The model under review builds one solid part; all positions refer to its coordinate system, in mm. A direction names the side the tool comes from. Round coordinates to 2 decimals unless told otherwise and drop trailing zeros. Write each loop counter-clockwise with the first axis right and the second up, starting at its lowest first coordinate (ties: lowest second). Pieces come first, ordered by that corner, then holes. Notation, with made-up numbers: (38.25, 8.5) - (85.25, 8.5) arc R32 cw to (85.25, 47.5) - close; hole circle Ø10 at (56.25, -1.75). An arc over 180 degrees is marked (long way). Write each question's results on one line, items separated by ' | '.
```python
from build123d import *

# Parameters (mm, degrees)
BOSS_EXTRUDE1_DEPTH = 15
SKETCH2_R           = 20
BOSS_EXTRUDE2_DEPTH = 25
SKETCH3_R           = 12.5
CUT_EXTRUDE1_DEPTH  = 103.220350224
SKETCH4_W           = 15
SKETCH4_H           = 65
BOSS_EXTRUDE3_DEPTH = 15


with BuildPart() as part:
    # Sketch1 → Boss-Extrude1 (new body)
    with BuildSketch(Plane.XY):
        with BuildLine():
            Line((0, 0), (68, 0))
            Line((68, 0), (68, 65))
            Line((68, 65), (0, 65))
            ThreePointArc((0, 65), (-32.5, 32.5), (0, 0))
        make_face()
    extrude(amount=BOSS_EXTRUDE1_DEPTH)

    # Sketch2 → Boss-Extrude2 (add)
    with BuildSketch(Plane.XY.offset(15)):
        with Locations((0, 32.5)):
            Circle(SKETCH2_R)
    extrude(amount=BOSS_EXTRUDE2_DEPTH)

    # Sketch3 → Cut-Extrude1 (cut, through all)
    with BuildSketch(Plane.XY.offset(40)):
        with Locations((0, 32.5)):
            Circle(SKETCH3_R)
    extrude(amount=-CUT_EXTRUDE1_DEPTH, mode=Mode.SUBTRACT)

    # Sketch4 → Boss-Extrude3 (add)
    with BuildSketch(Plane(origin=(0, 0, 0), x_dir=(-1, 0, 0), z_dir=(0, 0, -1))):
        with Locations((-60.5, 32.5)):
            Rectangle(SKETCH4_W, SKETCH4_H)
    extrude(amount=BOSS_EXTRUDE3_DEPTH)


solid = part.part
```
Q1. We need section D-D (y = 14). State the section outline as (x, z) points, plus the area to 3 significant figures.
Evaluation:
outline: (-26.72, 0) - (53, 0) - (53, -15) - (68, -15) - (68, 15) - (7.6, 15) - (7.6, 40) - (-7.6, 40) - (-7.6, 15) - (-26.72, 15) - close | area: 2,030 mm^2
Q2. Tool access review of faces 1 (the cylindrical face through (-32.492, 33.215, 7.395)), 2 (the cylindrical face through (-2.6, 52.33, 27.32)), 3 (the flat face through (53, 32, -7)): name each direction out of +Z, -Z, +X, -X, +Y, -Y from which nothing blocks a thin tool from reaching the whole face with its end or side.
Evaluation:
face 1: +Z, -Z, -X | face 2: +Z | face 3: -Z, -X, +Y, -Y
Q3. We need section A-A (y = 32.5). State the section outline as (x, z) points.
Evaluation:
outline: (-32.5, 0) - (-12.5, 0) - (-12.5, 40) - (-20, 40) - (-20, 15) - (-32.5, 15) - close; (12.5, 0) - (53, 0) - (53, -15) - (68, -15) - (68, 15) - (20, 15) - (20, 40) - (12.5, 40) - close
Q4. Insertion check: P1, Ø19.5, axis at x = -4.5, y = 26, coming from the +Z side; P2, Ø12, axis at x = 20, y = 12, coming from the +Z side; P3, Ø4, axis at y = 33, z = 20.5, coming from the -X side; P4, Ø2, axis at x = -19.5, y = 29.5, coming from the -Z side. Each pin has a flat end and moves straight along its axis. Give the tip position at first contact, or say it passes through.
Evaluation:
P1: stops at z = 40 | P2: stops at z = 15 | P3: stops at x = -20 | P4: stops at z = 0
Q5. We need section B-B (z = 10). State the section outline as (x, y) points, plus the area to 3 significant figures.
Evaluation:
outline: (0, 0) - (68, 0) - (68, 65) - (0, 65) arc R32.5 ccw to start; hole circle Ø25 at (0, 32.5) | area: 5,590 mm^2
Q6. For probe 1 along Y at (x, z) = (0, 17); probe 2 along X at (y, z) = (32, 17); probe 3 along Y at (x, z) = (0, 10), list the stretches that pass through material, from the lowest coordinate up.
Evaluation:
probe 1: y = 12.5 to 20, 45 to 52.5 | probe 2: x = -19.99 to -12.49, 12.49 to 19.99 | probe 3: y = 0 to 20, 45 to 65
Q7. We need section C-C (x = -14.5). State the section outline as (y, z) points.
Evaluation:
outline: (3.41, 0) - (61.59, 0) - (61.59, 15) - (46.27, 15) - (46.27, 40) - (18.73, 40) - (18.73, 15) - (3.41, 15) - close
